Design review of the part built by this model. Coordinates are the model's own, in mm. A direction names the side the tool comes from. Round coordinates to 2 decimals unless told otherwise and drop trailing zeros. Write each loop counter-clockwise with the first axis right and the second up, starting at its lowest first coordinate (ties: lowest second). Pieces come first, ordered by that corner, then holes. Notation, with made-up numbers: M 43,71 L 92,71 A21 ccw 92,76 Z; hole C 68,8.5 d5. An arc over 180 degrees is marked long. Use CSV: the item, a comma, the result in double quotes.
from build123d import *

# Parameters (mm, degrees)
SKIZZE1_W                             = 15
SKIZZE1_H                             = 20
AUFSATZ_LINEAR_AUSTRAGEN8_DEPTH       = 30
AUFSATZ_LINEAR_AUSTRAGEN10_DEPTH      = 3
AUFSATZ_LINEAR_AUSTRAGEN10_DEPTH_BACK = 18
SKIZZE2_R                             = 5


with BuildPart() as part:
    # Skizze1 → Aufsatz-Linear austragen8 (new body)
    with BuildSketch(Plane.XY):
        with Locations((7.5, 10)):
            Rectangle(SKIZZE1_W, SKIZZE1_H)
    extrude(amount=AUFSATZ_LINEAR_AUSTRAGEN8_DEPTH)

    # Skizze2 → Aufsatz-Linear austragen10 (add, two sides: drawn at the far end of the back side and taken through both)
    with BuildSketch(Plane(origin=(15, 0, 0), x_dir=(0, 0, -1), z_dir=(1, 0, 0)).offset(-AUFSATZ_LINEAR_AUSTRAGEN10_DEPTH_BACK)):
        with Locations((-22, 10)):
            Circle(SKIZZE2_R)
    extrude(amount=AUFSATZ_LINEAR_AUSTRAGEN10_DEPTH + AUFSATZ_LINEAR_AUSTRAGEN10_DEPTH_BACK)


with BuildPart() as part_1:
    # Körper-Verschieben/Kopieren1: moved
    add(part.part.moved(Location((3, 0, 0))))


solid = part_1.part
1) Wall thickness on line 1 along X through (y, z) = (7, 27.5); line 2 along Z through (x, y) = (18.5, 11.75): over which ranges is each line inside the solid? List them lowest first. Write a range as [from, to].
Answers:
line 1,"[3, 18]"
line 2,"[17.32, 26.68]"
2) Add section B-B on y = 10. Write out the cut boundary in (x, z).
Answers:
outline,"M 0,17 L 3,17 L 3,0 L 18,0 L 18,17 L 21,17 L 21,27 L 18,27 L 18,30 L 3,30 L 3,27 L 0,27 Z"
3) Add section A-A on z = 22. Write out the cut boundary in (x, y), then the cut area to 3 significant figures.
Answers:
outline,"M 0,5 L 3,5 L 3,0 L 18,0 L 18,5 L 21,5 L 21,15 L 18,15 L 18,20 L 3,20 L 3,15 L 0,15 Z"
area,"360 mm²"
4) Machinability: for faces 1 (the face through (19, 10, 27)), 2 (the face through (21, 10, 22)), 3 (the face through (1, 10, 27)), which of the approach directions +Z, -Z, +X, -X, +Y, -Y give a long, thin tool a straight path to every point of the face, cutting with its end or side? Answer none if there is none.
Answers:
face 1,"+X"
face 2,"+Z, -Z, +X, +Y, -Y"
face 3,"-X"
5) For pin 1 Ø5 at (y, z) = (7.5, 9.5) entering from -X; pin 2 Ø10 at (y, z) = (5.5, 7.5) entering from +X, all flat-tipped, find the tip position at first contact; note any pin that passes through.
Answers:
pin 1,"x = 3"
pin 2,"x = 18"
6) Add section C-C on y = 16.75. Write out the cut boundary in (x, z), then the cut area to 3 significant figures.
Answers:
outline,"M 3,0 L 18,0 L 18,30 L 3,30 Z"
area,"450 mm²"
